Geometry check sheet. Reference: the model listing, model coordinates, mm. Face numbers are marked on the shaded views. A direction names the side the tool comes from. Give positions to 0.01 mm unless a question says otherwise; leave off trailing zeros. Write each loop counter-clockwise with the first axis right and the second up, starting at its lowest first coordinate (ties: lowest second). Pieces come first, ordered by that corner, then holes. Notation, with made-up numbers: (39, -3.75) - (85, -3.75) arc R25 cw to (85, 9.25) - close; hole circle Ø1 at (-34.75, 89). An arc over 180 degrees is marked (long way). Use a Markdown table: item, result.
```python
from build123d import *

# Parameters (mm, degrees)
SKETCH1_R          = 23.8125
EXTRUDE1_DEPTH     = 53.848
CHAMFER1_SIZE      = 0.762
SKETCH6_R          = 22.225
EXTRUDE2_DEPTH     = 5.969
SKETCH7_W          = 16.51
SKETCH7_H          = 14.2875
CUT_EXTRUDE4_DEPTH = 19.84248
HOLE1_D            = 5.0038
HOLE1_DEPTH        = 4.7498
CIRPATTERN1_COUNT  = 4


with BuildPart() as part:
    # Sketch1 → Extrude1 (new body)
    with BuildSketch(Plane.XY):
        Circle(SKETCH1_R)
    extrude(amount=EXTRUDE1_DEPTH)

    # Sketch2 → Cut-Revolve1 (revolve, cut)
    with BuildSketch(Plane(origin=(0, 0, 0), x_dir=(1, 0, 0), z_dir=(0, 1, 0)), mode=Mode.PRIVATE) as cut_revolve1_sk:
        Polygon((23.8125, -53.848), (23.8125, -39.751), (22.4155, -41.148), (22.4155, -53.848), align=None)
    revolve(cut_revolve1_sk.sketch.rotate(Axis((0, 0, 0), (0, 0, 1)), 180), axis=Axis((0, 0, 0), (0, 0, 1)), mode=Mode.SUBTRACT)  # turned: the seam where the file's is

    # Sketch3 → Cut-Revolve2 (revolve, cut)
    with BuildSketch(Plane(origin=(0, 0, 0), x_dir=(1, 0, 0), z_dir=(0, 1, 0)), mode=Mode.PRIVATE) as cut_revolve2_sk:
        Polygon((22.4155, 0), (22.4155, -1.524), (23.8125, -2.921), (23.8125, 0), align=None)
    revolve(cut_revolve2_sk.sketch.rotate(Axis((0, 0, 0), (0, 0, -1)), 180), axis=Axis((0, 0, 0), (0, 0, -1)), mode=Mode.SUBTRACT)  # turned: the seam where the file's is

    # S2D0002 → Cut-Revolve3 (revolve, cut)
    with BuildSketch(Plane(origin=(0, 0, 0), x_dir=(1, 0, 0), z_dir=(0, 1, 0))):
        Polygon((6.1849, -53.594), (9.525, -53.594), (9.525, -53.848), (0, -53.848), (0, -39.624), (4.9784, -39.624), (4.9784, -50.377393135), (5.642306865, -51.0413), align=None)
    revolve(axis=Axis((0, 0, 14.6685), (0, 0, -1)), mode=Mode.SUBTRACT)

    # Chamfer1
    chamfer1_edges = [part.edges().sort_by_distance(p)[0] for p in [
        (22.4155, 0, 53.848),
    ]]
    chamfer(chamfer1_edges, length=CHAMFER1_SIZE)

    # Sketch6 → Extrude2 (add)
    with BuildSketch(Plane(origin=(0, 0, 0), x_dir=(-1, 0, 0), z_dir=(0, 0, -1))):
        with Locations(Location((0, 0, 0), (0, 0, 180))):  # turned: the seam where the file's is
            Circle(SKETCH6_R)
    extrude(amount=EXTRUDE2_DEPTH)

    # Sketch7 → Revolve1 (revolve)
    with BuildSketch(Plane(origin=(0, 0, 0), x_dir=(0, 0, -1), z_dir=(1, 0, 0)), mode=Mode.PRIVATE) as revolve1_sk:
        with Locations((14.224, -7.14375)):
            Rectangle(SKETCH7_W, SKETCH7_H)
    revolve(revolve1_sk.sketch.rotate(Axis((0, 0, 0), (0, 0, -1)), 270), axis=Axis((0, 0, 0), (0, 0, -1)))  # turned: the seam where the file's is

    # S2D0001 → Cut-Revolve5 (revolve, cut)
    with BuildSketch(Plane(origin=(0, 0, 0), x_dir=(1, 0, 0), z_dir=(0, 1, 0))):
        Polygon((5.5499, 20.411277746), (5.5499, 3.8608), (0, 3.8608), (0, 22.479), (6.7437, 22.479), align=None)
    revolve(axis=Axis((0, 0, 31.308359971), (0, 0, -1)), mode=Mode.SUBTRACT)

    # Sketch9 → Cut-Revolve6 (revolve, cut)
    with BuildSketch(Plane(origin=(0, 0, 0), x_dir=(0, -1, 0), z_dir=(1, 0, 0)), mode=Mode.PRIVATE) as cut_revolve6_sk:
        with BuildLine():
            Line((-14.2875, 12.573), (-14.097, 13.335))
            Line((-14.097, 13.335), (-14.097, 21.463))
            ThreePointArc((-14.097, 21.463), (-13.996678675, 22.006796865), (-13.708922533, 22.479))
            Line((-13.708922533, 22.479), (-14.2875, 22.479))
            Line((-14.2875, 22.479), (-14.2875, 12.573))
        make_face()
    revolve(cut_revolve6_sk.sketch.rotate(Axis((0, 0, -12.65936), (0, 0, -1)), 90), axis=Axis((0, 0, -12.65936), (0, 0, -1)), mode=Mode.SUBTRACT)  # turned: the seam where the file's is

    # Sketch13 → Cut-Extrude4 (cut, symmetric)
    with BuildSketch(Plane(origin=(0, 0, 0), x_dir=(1, 0, 0), z_dir=(0, 1, 0))):
        Polygon((12.573, 22.479), (12.573, 14.9098), (14.2875, 13.1953), (14.2875, 22.479), align=None)
        Polygon((-12.573, 22.479), (-12.573, 14.9098), (-14.2875, 13.1953), (-14.2875, 22.479), align=None)
    extrude(amount=CUT_EXTRUDE4_DEPTH, both=True, mode=Mode.SUBTRACT)

    # Hole1
    with Locations(Plane(origin=(-15.850152054, 15.850152054, 47.498), x_dir=(0.707106781, 0.707106781, 0), z_dir=(-0.707106781, 0.707106781, 0))):
        with Locations((0, 0)):
            hole1 = Hole(HOLE1_D / 2, depth=HOLE1_DEPTH)

    # CirPattern1: Hole1 ×4 about axis
    cirpattern1_axis = Axis((0, 0, 0), (0, 0, 1))
    for i in range(1, CIRPATTERN1_COUNT):
        add(hole1.rotate(cirpattern1_axis, i * 360 / CIRPATTERN1_COUNT), mode=Mode.SUBTRACT)


solid = part.part
```
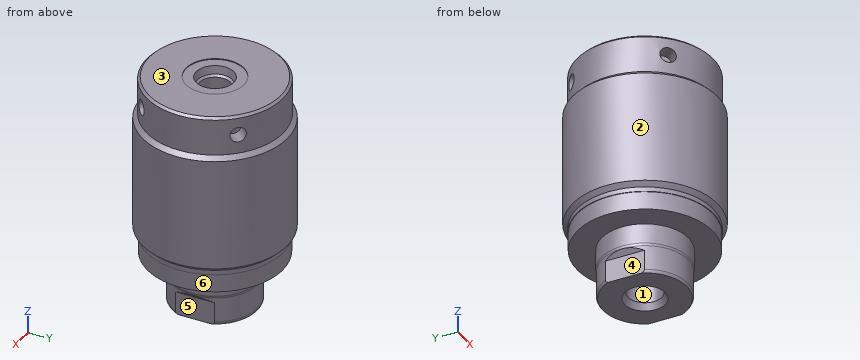
1) Material ranges on L1, parallel to X at y = 0, z = -17; L2, parallel to Z at x = 3.5, y = 17; L3, parallel to Z at x = -14, y = 12, recorded low to high. Write a range as from..to.
Working result:
| item | result |
|---|---|
| L1 | x = -12.57..-5.55, 5.55..12.57 |
| L2 | z = -5.97..53.85 |
| L3 | z = -5.97..45.43, 49.56..53.85 |
2) Section check B-B on z = 33.5. Record the boundary of the cut face in (x, y) (1 decimal), then the cut area to 3 significant figures.
Working result:
| item | result |
|---|---|
| outline | circle Ø47.6 at (0, 0) |
| area | 1,780 mm² |
3) Mould release check, pull along Y, two halves, no side actions. Record for the marked faces 1, 2 and 3: pulls with the +Y half, pulls with the -Y half, needs draft (parallel to the pull), parting line crosses it, or undercut.
Working result:
| item | result |
|---|---|
| face 1 | undercut |
| face 2 | parting line crosses it |
| face 3 | needs draft |
4) Set-up check for the marked faces 4, 5 and 6: record each of +Z, -Z, +X, -X, +Y, -Y from which the full face is reachable in a straight line by a thin tool's end or side.
Working result:
| item | result |
|---|---|
| face 4 | -Z, -X, +Y, -Y |
| face 5 | -Z, +X, +Y, -Y |
| face 6 | -Z |
5) Section check A-A on z = -17. Record the boundary of the cut face in (x, y), then the cut area to 3 significant figures.
Working result:
| item | result |
|---|---|
| outline | (-12.57, -6.38) arc R14.1 ccw to (12.57, -6.38) - (12.57, 6.38) arc R14.1 ccw to (-12.57, 6.38) - close; hole circle Ø11.1 at (0, 0) |
| area | 501 mm² |
6) Depth check by flat-ended pin: P1, Ø3, axis at y = 0, z = 44.5, coming from the +X side; P2, Ø14.5, axis at x = 0, y = 0, coming from the +Z side; P3, Ø6, axis at x = -10, z = 30.5, coming from the +Y side. Enter the tip coordinate at first touch or a pass-through.
Working result:
| item | result |
|---|---|
| P1 | stops at x = 22.42 |
| P2 | stops at z = 53.59 |
| P3 | stops at y = 22.76 |
